from build123d import *

# Parameters (mm, degrees)
F0_W        = 81.7
F0_H        = 129.7
F0_W_2      = 79.3
F0_H_2      = 127.3
F1_DEPTH    = 5.5
F1_FACE_W   = 81.7
F1_FACE_H   = 129.7
F1_FACE_W_2 = 79.3
F1_FACE_H_2 = 127.3
F2_DEPTH    = 1.2
F3_R        = 2.5
F4_R        = 2


with BuildPart() as f1:
    # F0 (on Top) → F1 (new body)
    with BuildSketch(Plane.XY):
        with Locations((-7.4785080035, 23.4226425927)):
            Rectangle(F0_W, F0_H)
        with Locations((-7.4785080035, 23.4226425927)):
            Rectangle(F0_W_2, F0_H_2, mode=Mode.SUBTRACT)
    extrude(amount=F1_DEPTH)

    # F0 (on Top) + F1_face (on face) → F2 (join)
    with BuildSketch(Plane.XY):
        with Locations((-7.4785080035, 23.4226425927)):
            Rectangle(F0_W_2, F0_H_2)
    with BuildSketch(Plane(origin=(-7.4785080035, 23.4226425927, 0), x_dir=(1, 0, 0), z_dir=(0, 0, -1))):
        Rectangle(F1_FACE_W, F1_FACE_H)
        Rectangle(F1_FACE_W_2, F1_FACE_H_2, mode=Mode.SUBTRACT)
    extrude(amount=-F2_DEPTH, dir=(0, 0, 1))

    # F3
    f3_edges = [f1.edges().sort_by_distance(p)[0] for p in [
        (-48.328508, 88.272643, 2.15),
        (-48.328508, -41.427357, 2.15),
        (33.371492, -41.427357, 2.15),
        (33.371492, 88.272643, 2.15),
    ]]
    fillet(f3_edges, radius=F3_R)

    # F4
    f4_edges = [f1.edges().sort_by_distance(p)[0] for p in [
        (-7.478508, 88.272643, -1.2),
        (-47.596275, 87.54041, -1.2),
        (32.639259, 87.54041, -1.2),
        (-48.328508, 23.422643, -1.2),
        (33.371492, 23.422643, -1.2),
        (-47.596275, -40.695124, -1.2),
        (32.639259, -40.695124, -1.2),
        (-7.478508, -41.427357, -1.2),
    ]]
    fillet(f4_edges, radius=F4_R)


solid = f1.part
Part model, mm, in its own coordinate system. A direction names the side the tool comes from. Coordinates: 2 decimals unless noted, no trailing zeros. Write each loop counter-clockwise with the first axis right and the second up, starting at its lowest first coordinate (ties: lowest second). Pieces come first, ordered by that corner, then holes. Notation, with made-up numbers: M 39.5,63.25 L 78.5,63.25 A20 ccw 78.5,78.25 Z; hole C 78,-34 d4. An arc over 180 degrees is marked long. Return JSON: item names as keys, results as strings.
1. Probe L1, parallel to Y at x = 6, z = 3; L2, parallel to X at y = 40.5, z = 2.25; L3, parallel to X at y = -35, z = 0.5. List the from-to ranges inside material, lowest first.
Determined:
{"L1": "-41.43 to -40.23, 87.07 to 88.27", "L2": "-48.33 to -47.13, 32.17 to 33.37", "L3": "-48.31 to -47.13, 32.17 to 33.35"}
2. Flat gauge pin, fed straight in: pin 1 Ø8 at (x, y) = (14, 0) entering from +Z. Where does the tip first touch, or does it go through?
Determined:
{"pin 1": "z = 0"}
3. Saw through at A-A, the plane z = 3.25. Write the cut outline in (x, y).
Determined:
{"outline": "M -48.33,-38.93 A2.5 ccw -45.83,-41.43 L 30.87,-41.43 A2.5 ccw 33.37,-38.93 L 33.37,85.77 A2.5 ccw 30.87,88.27 L -45.83,88.27 A2.5 ccw -48.33,85.77 Z; hole M -47.13,-40.23 L 32.17,-40.23 L 32.17,87.07 L -47.13,87.07 Z"}
4. 3-axis set-ups, long thin cutter, end or side, ignore diameter. For faces 5 (the face through (-47.129, 23, 3)), 6 (the face through (-47.577, 87.56, 3.117)): which of +Z, -Z, +X, -X, +Y, -Y reach the whole face in a straight line?
Determined:
{"face 5": "+Z", "face 6": "+Z, -Z, -X, +Y"}
5. Pull direction X, two halves, no side cores. Call faces 1 (the face through (-8, -41.427, 3)), 2 (the face through (-8, 24, 0)), 3 (the face through (-48.329, 23, 3)), 4 (the face through (33.371, 23, 3)): pulls with the +X half, pulls with the -X half, needs draft (parallel to the pull), parting line crosses it, or undercut.
Determined:
{"face 1": "needs draft", "face 2": "undercut", "face 3": "pulls with the -X half", "face 4": "pulls with the +X half"}
6. Saw through at B-B, the plane y = 56.5. Write the cut outline in (x, z).
Determined:
{"outline": "M -48.33,0.8 A2 ccw -46.33,-1.2 L 31.37,-1.2 A2 ccw 33.37,0.8 L 33.37,5.5 L 32.17,5.5 L 32.17,0 L -47.13,0 L -47.13,5.5 L -48.33,5.5 Z"}
7. Saw through at C-C, the plane x = -11. Write the cut outline in (y, z).
Determined:
{"outline": "M -41.43,0.8 A2 ccw -39.43,-1.2 L 86.27,-1.2 A2 ccw 88.27,0.8 L 88.27,5.5 L 87.07,5.5 L 87.07,0 L -40.23,0 L -40.23,5.5 L -41.43,5.5 Z"}
